from build123d import *

# Parameters (mm, degrees)
SKETCH2_R          = 4.5
CUT_EXTRUDE1_DEPTH = 50


with BuildPart() as part:
    # Sketch1 → Base-Revolve (revolve)
    with BuildSketch(Plane.XY):
        with BuildLine():
            Line((0, 21), (0, 23.5))
            Line((0, 23.5), (0.5, 24))
            Line((0.5, 24), (5, 24))
            Line((5, 24), (5, 24.75))
            Line((5, 24.75), (13, 24.75))
            Line((13, 24.75), (13, 25))
            Line((13, 25), (2230.5, 25))
            Line((2230.5, 25), (2232, 24.133974596))
            Line((2232, 24.133974596), (2232, 23.8))
            ThreePointArc((2232, 23.8), (2232.234314575, 23.234314575), (2232.8, 23))
            Line((2232.8, 23), (2237.2, 23))
            ThreePointArc((2237.2, 23), (2237.765685425, 23.234314575), (2238, 23.8))
            Line((2238, 23.8), (2238, 24.25))
            ThreePointArc((2238, 24.25), (2238.146446609, 24.603553391), (2238.5, 24.75))
            Line((2238.5, 24.75), (2239.5, 24.75))
            Line((2239.5, 24.75), (2241, 23.883974596))
            Line((2241, 23.883974596), (2241, 23.55))
            ThreePointArc((2241, 23.55), (2241.234314575, 22.984314575), (2241.8, 22.75))
            Line((2241.8, 22.75), (2244, 22.75))
            Line((2244, 22.75), (2246.453263132, 24))
            Line((2246.453263132, 24), (2270.401923789, 24))
            Line((2270.401923789, 24), (2273, 22.5))
            Line((2273, 22.5), (2283, 22.5))
            Line((2283, 22.5), (2284, 21.922649731))
            Line((2284, 21.922649731), (2284, 17))
            Line((2284, 17), (6.92820323, 17))
            Line((6.92820323, 17), (0, 21))
        make_face()
    revolve(axis=Axis((0, 0, 0), (1, 0, 0)))

    # Sketch2 → Cut-Extrude1 (cut, symmetric)
    with BuildSketch(Plane.XY):
        with Locations((2220, 0)):
            Circle(SKETCH2_R)
    extrude(amount=CUT_EXTRUDE1_DEPTH, both=True, mode=Mode.SUBTRACT)


solid = part.part
Source: CAD feature listing. Evaluate the final solid. Frame: model axes, mm. A direction names the side the tool comes from. Round coordinates to 2 decimals unless told otherwise and drop trailing zeros. Loops run counter-clockwise (first coordinate to the right, second up) from the corner with the lowest first, then second, coordinate; pieces in that order, holes last. Notation, with made-up numbers: (32.25, 28.25) -> (57.25, 28.25) arc R16 ccw to (57.25, 32.25) -> close; hole circle Ø11 at (82.5, 4.25). An arc over 180 degrees is marked (long way). Answer as a JSON object with one key per item and string values. Group by question number.
Q1. Contact query for flat-ended pins moving along their axis: P1, Ø8, axis at y = -14, z = 17.5, coming from the -X side; P2, Ø14.5, axis at y = -12, z = -6, coming from the -X side; P3, Ø14.5, axis at y = -7, z = 0.5, coming from the +X side; P4, Ø5, axis at x = 1876.5, z = -12, coming from the +Y side. Output: stop coordinate, or through.
Q2. Section query A-A (x = 351.5). Output: boundary loops of the cut face in (y, z), plus the area to 3 significant figures.
Q3. Access query for faces 1 (the flat face through (2238, -18, -16)), 2 (the flat face through (5, 4, 24)). Directions: +Z, -Z, +X, -X, +Y, -Y. A direction counts if a zero-diameter tool reaches every point of the face in a straight line with its end or side. Return the directions, or none.
Q4. Mould query, pull axis Y, two halves, no side actions, for faces 3 (the conical face through (6.495, 16.454, 5.181)), 4 (the flat face through (2241, 11, -21)), 5 (the cylindrical face through (2239.01, -3.22, 24.54)). Classes: pulls with the +Y half, pulls with the -Y half, needs draft (parallel to the pull), parting line crosses it, or undercut.
Q5. Ray query, line 1 (Y direction, x = 1247, z = 1); line 2 (X direction, y = 0, z = 21.25); line 3 (Z direction, x = 1031, y = -3). Return the intervals inside material, ascending. Write a range as from..to.
Completed:
{
 "1": {"P1": "x = 0", "P2": "x = 0.58", "P3": "through", "P4": "y = 23.12"},
 "2": {"outline": "circle Ø50 at (0, 0); hole circle Ø34 at (0, 0)", "area": "1,060 mm²"},
 "3": {"face 1": "none", "face 2": "-X"},
 "4": {"face 3": "undercut", "face 4": "needs draft", "face 5": "parting line crosses it"},
 "5": {"line 1": "-24.98..-16.97, 16.97..24.98", "line 2": "0..2215.5, 2224.5..2284", "line 3": "-24.82..-16.73, 16.73..24.82"}
}
